from build123d import *

# Parameters (mm, degrees)
SKETCH2_R               = 2.35
BOSS_EXTRUDE1_DEPTH     = 15
CUT_EXTRUDE2_DEPTH      = 25
CUT_EXTRUDE2_DEPTH_BACK = 25


with BuildPart() as part:
    # Sketch1 → Revolve2 (revolve)
    with BuildSketch(Plane.XY, mode=Mode.PRIVATE) as revolve2_sk:
        with BuildLine():
            Line((0, 27.986111111), (0, -7.013888889))
            Line((0, -7.013888889), (0, -22.013888889))
            ThreePointArc((0, -22.013888889), (10.606601718, -17.620490607), (15, -7.013888889))
            add(Edge.make_bspline(
                [(2.35, 27.986111111), (2.599847264, 21.390422987), (1.849692868, 12.096697956), (15.855089794, 0.539943119), (15, -7.013888889)],
                knots=[0, 0, 0, 0, 0.452531855, 1, 1, 1, 1], degree=3))
            Line((2.35, 27.986111111), (0, 27.986111111))
        make_face()
    revolve(revolve2_sk.sketch.rotate(Axis((0, 27.986111111, 0), (0, -1, 0)), 180), axis=Axis((0, 27.986111111, 0), (0, -1, 0)))  # turned: the seam where the file's is

    # Sketch2 → Boss-Extrude1 (add)
    with BuildSketch(Plane(origin=(0, 27.986111111, 0), x_dir=(1, 0, 0), z_dir=(0, 1, 0))):
        with Locations(Location((0, 0, 0), (0, 0, 180))):  # turned: the seam where the file's is
            Circle(SKETCH2_R)
    extrude(amount=BOSS_EXTRUDE1_DEPTH)

    # Sketch3 → Cut-Extrude2 (cut, two sides)
    with BuildSketch(Plane.XY) as cut_extrude2_sk:
        Polygon((0, 42.986111111), (0, 27.986111111), (0, -22.013888889), (0, -24.288490859), (33.029158628, -24.288490859), (33.029158628, 42.986111111), align=None)
    extrude(amount=CUT_EXTRUDE2_DEPTH, mode=Mode.SUBTRACT)
    extrude(cut_extrude2_sk.sketch, amount=-CUT_EXTRUDE2_DEPTH_BACK, mode=Mode.SUBTRACT)


solid = part.part
CAD build for the part. Positions are in the model's coordinates, mm. A direction names the side the tool comes from. Coordinates: 2 decimals unless noted, no trailing zeros. Loops run counter-clockwise (first coordinate to the right, second up) from the corner with the lowest first, then second, coordinate; pieces in that order, holes last. Notation, with made-up numbers: (52, -30.5) -> (94, -30.5) arc R31 ccw to (94, -5.5) -> close; hole circle Ø11 at (11, -24). An arc over 180 degrees is marked (long way). One line per item, written item: value.
1. Flat gauge pins, fed straight in: P1, Ø2, axis at y = -8, z = -11.5, coming from the -X side; P2, Ø4, axis at x = -3, z = -8.5, coming from the -Y side; P3, Ø3, axis at x = -3.5, y = 4.5, coming from the +Z side. Where does each tip first touch, or does it go through?
Answers:
P1: stops at x = -10.67
P2: stops at y = -20.27
P3: stops at z = 11.38
2. Drill centre lines: line 1 (X direction, y = -10, z = 6); line 2 (Y direction, x = -4.25, z = 2); line 3 (Y direction, x = -3.5, z = 6). Where is each one in solid material? Low to high. Write a range as [from, to].
Answers:
line 1: x = [-13.42, 0]
line 2: y = [-21.26, 12.96]
line 3: y = [-20.31, 9.53]
3. Slice it at A-A on y = 37. Write the cut outline in (x, z).
Answers:
outline: (0, -2.35) -> (0, 2.35) arc R2.35 ccw to start
4. Slice it at B-B on y = -15.5. Write the cut outline in (x, z), and give its area (3 significant figures).
Answers:
outline: (0, -12.37) -> (0, 12.37) arc R12.37 ccw to start
area: 240 mm^2
5. Which spindle directions (+Z, -Z, +X, -X, +Y, -Y) get a long thin tool onto all of the face, cutting with end or side? Do faces 1 (the face through (0, -4, 0)), 2 (the face through (-2.35, 35.38, -0.05)). Say none if no direction does.
Answers:
face 1: +Z, -Z, +X, +Y, -Y
face 2: -X, +Y
